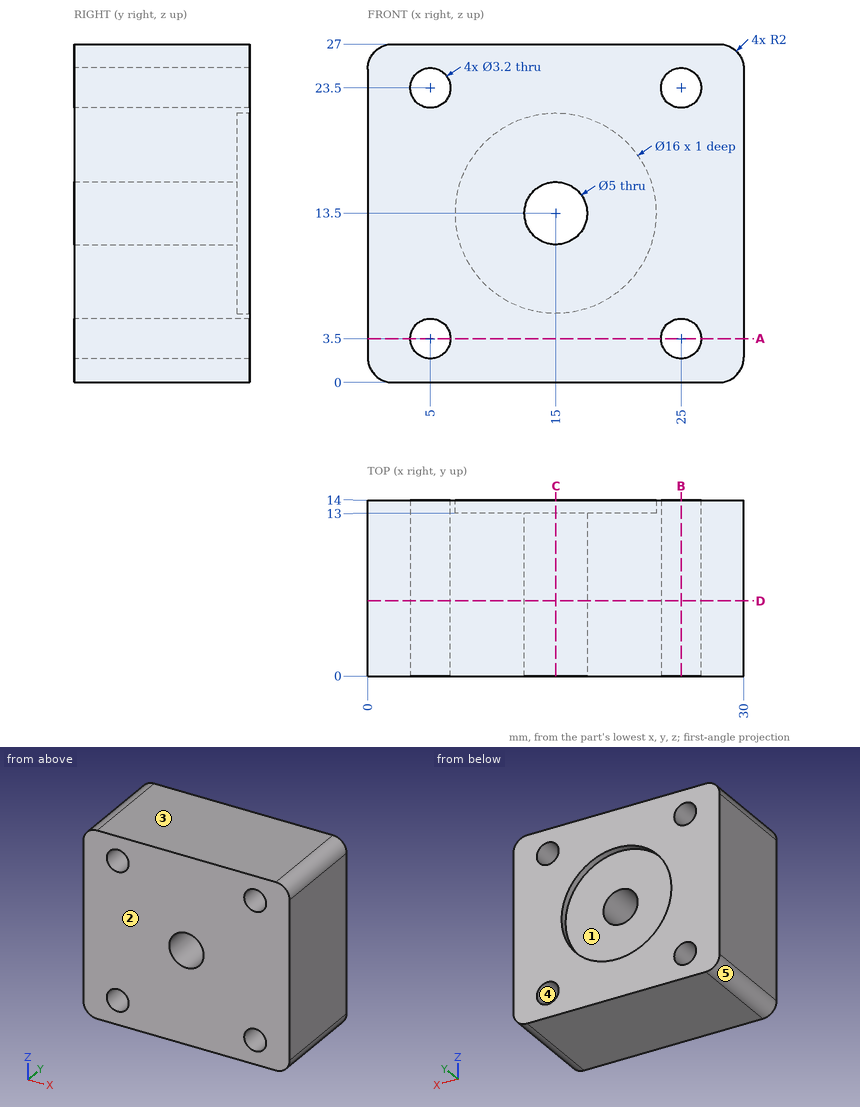
Design review of the part shown in the three views and the two pictorial views. Dimensions are in mm from the part's minimum x, y and z. A direction names the side the tool comes from. Give positions to 0.01 mm unless a question says otherwise; leave off trailing zeros. Write each loop counter-clockwise with the first axis right and the second up, starting at its lowest first coordinate (ties: lowest second). Pieces come first, ordered by that corner, then holes.
(1) Tool access review of the marked faces 1 and 2: name each direction out of +Z, -Z, +X, -X, +Y, -Y from which nothing blocks a thin tool from reaching the whole face with its end or side.
Checked values:
face 1: +Y
face 2: +Z, -Z, +X, -X, -Y
(2) Add section D-D (y = 6). Give the boundary of the cut face in (x, z), and give its area (3 significant figures).
Checked values:
outline: (0, 2) arc R2 ccw to (2, 0) - (28, 0) arc R2 ccw to (30, 2) - (30, 25) arc R2 ccw to (28, 27) - (2, 27) arc R2 ccw to (0, 25) - close; hole circle Ø3.2 at (5, 3.5); hole circle Ø3.2 at (5, 23.5); hole circle Ø5 at (15, 13.5); hole circle Ø3.2 at (25, 3.5); hole circle Ø3.2 at (25, 23.5)
area: 755 mm2
(3) Wall thickness on line 1 along X through (y, z) = (7, 23.5); line 2 along Z through (x, y) = (5, 7.25); line 3 along Z through (x, y) = (23.75, 10): over which ranges is each line inside the solid? List them lowest first.
Checked values:
line 1: x = 0 to 3.4, 6.6 to 23.4, 26.6 to 30
line 2: z = 0 to 1.9, 5.1 to 21.9, 25.1 to 27
line 3: z = 0 to 2.5, 4.5 to 22.5, 24.5 to 27
(4) Mouldability with a two-part tool opening along X and no side actions: class the marked faces 3, 4 and 5 as +X half, -X half, draft (parallel to the pull), parting line (faces both ways), or undercut.
Checked values:
face 3: draft
face 4: undercut
face 5: -X half
(5) Add section C-C (x = 15). Give the boundary of the cut face in (y, z), and give its area (3 significant figures).
Checked values:
outline: (0, 0) - (14, 0) - (14, 5.5) - (13, 5.5) - (13, 11) - (0, 11) - close; (0, 16) - (13, 16) - (13, 21.5) - (14, 21.5) - (14, 27) - (0, 27) - close
area: 297 mm2
(6) Add section B-B (x = 25). Give the boundary of the cut face in (y, z).
Checked values:
outline: (0, 0) - (14, 0) - (14, 1.9) - (0, 1.9) - close; (0, 5.1) - (14, 5.1) - (14, 21.9) - (0, 21.9) - close; (0, 25.1) - (14, 25.1) - (14, 27) - (0, 27) - close
(7) Add section A-A (z = 3.5). Give the boundary of the cut face in (x, y).
Checked values:
outline: (0, 0) - (3.4, 0) - (3.4, 14) - (0, 14) - close; (6.6, 0) - (23.4, 0) - (23.4, 14) - (6.6, 14) - close; (26.6, 0) - (30, 0) - (30, 14) - (26.6, 14) - close
(8) Clearance check with flat-ended pins moving along their axes: pin 1 Ø4.5 at (x, z) = (15, 13.5) entering from +Y; pin 2 Ø8 at (x, z) = (18.5, 14) entering from +Y. State where each tip first meets the part, or that it passes through.
Checked values:
pin 1: passes through
pin 2: stops at y = 13
